Geometry: see drawing. Coordinates: mm, zero at the bounding-box minimum. Coordinates: 2 decimals unless noted, no trailing zeros. Order: outer loops, then holes, each group sorted by start corner. A loop starts at its lowest first (then second) coordinate and runs counter-clockwise, first axis right, second up. Notation, with made-up numbers: (47, 89) -> (52, 89) arc R30 ccw to (52, 122) -> close; hole circle Ø8 at (42, 49.5). An arc over 180 degrees is marked (long way). Use one line per item in the form item = value.
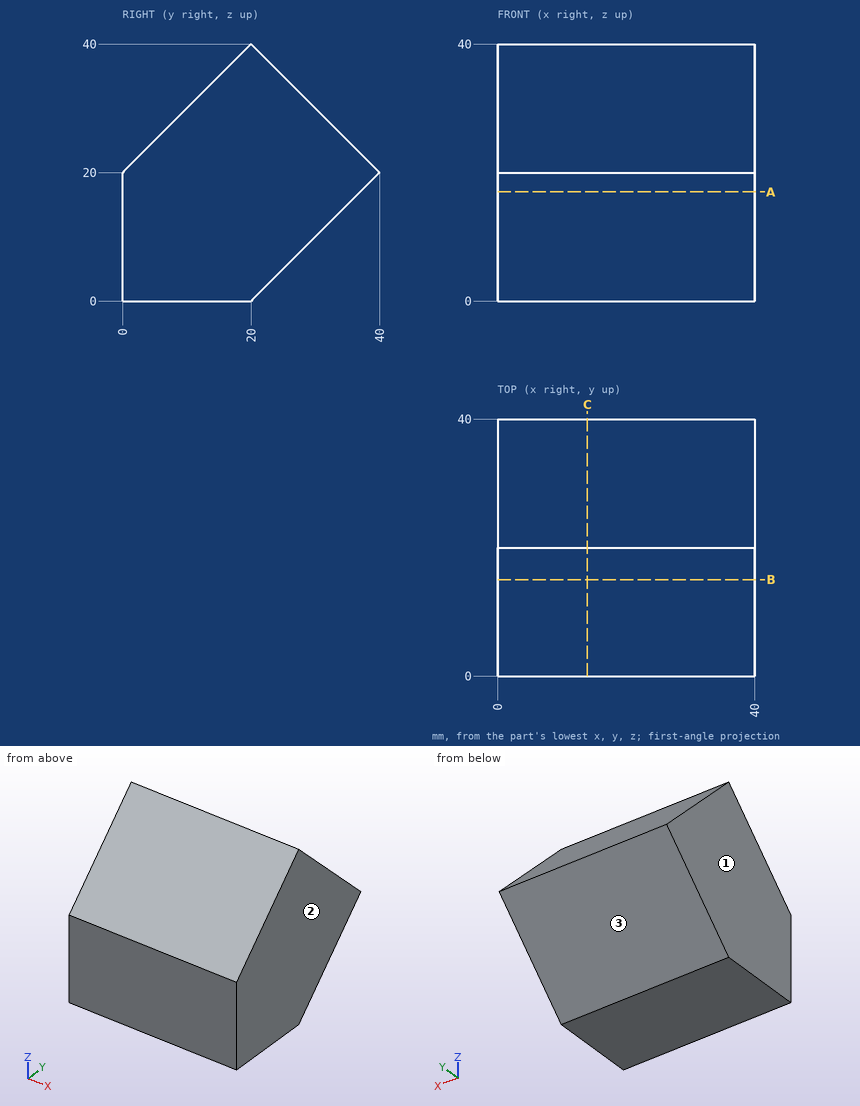
1) Section B-B, the plane y = 15. Output: boundary loops of the cut face in (x, z).
Results found:
outline = (0, 0) -> (40, 0) -> (40, 35) -> (0, 35) -> close
2) Material intervals for probe 1 along Y at (x, z) = (10, 35.5); probe 2 along Z at (x, y) = (27, 25); probe 3 along Y at (x, z) = (20, 33.5), sorted ascending. Write a range as from..to.
Results found:
probe_1 = 15.5..24.5
probe_2 = 5..35
probe_3 = 13.5..26.5
3) Pull-direction query (X, two-part tool) for the marked faces 1, 2 and 3; classes: released by +X, released by -X, zero draft, split by the parting line, or undercut.
Results found:
face_1 = released by -X
face_2 = released by +X
face_3 = zero draft
4) Section A-A, the plane z = 17. Output: boundary loops of the cut face in (x, y), and give its area (3 significant figures).
Results found:
outline = (0, 0) -> (40, 0) -> (40, 37) -> (0, 37) -> close
area = 1,480 mm2
5) Section C-C, the plane x = 14. Output: boundary loops of the cut face in (y, z).
Results found:
outline = (0, 0) -> (20, 0) -> (40, 20) -> (20, 40) -> (0, 20) -> close
6) Contact query for flat-ended pins moving along their axis: P1, Ø6, axis at y = 34.5, z = 12.5, coming from the -X side; P2, Ø6, axis at x = 18.5, z = 33.5, coming from the -Y side; P3, Ø3, axis at x = 30, y = 4.5, coming from the +Z side; P4, Ø5, axis at x = 11, y = 14.5, coming from the +Z side. Output: stop coordinate, or through.
Results found:
P1 = 0
P2 = 10.5
P3 = 26
P4 = 37
